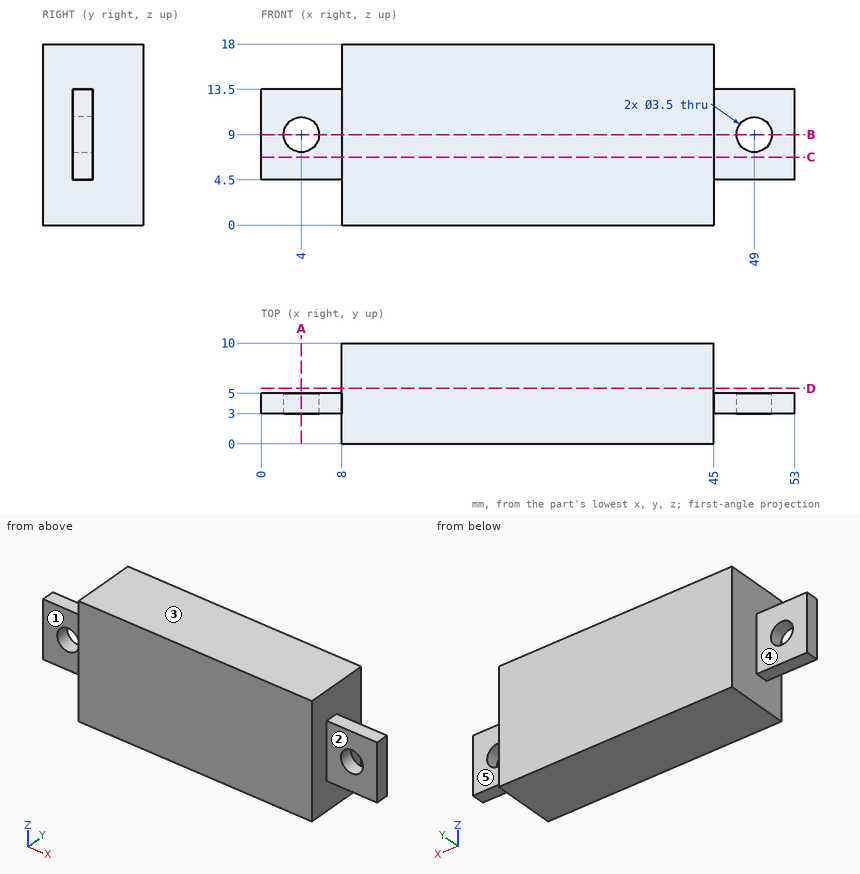
Check sheet for the drawn part. Datum: minimum x, y, z corner. Units: mm. A direction names the side the tool comes from. Give positions to 0.01 mm unless a question says otherwise; leave off trailing zeros. Loops run counter-clockwise (first coordinate to the right, second up) from the corner with the lowest first, then second, coordinate; pieces in that order, holes last.
1) Sectioned sample at A-A, the plane x = 4. Enter the section's corners in (y, z).
2) Depth check by flat-ended pin: pin 1 Ø5 at (y, z) = (3.5, 6) entering from -X; pin 2 Ø2 at (y, z) = (9, 13.5) entering from +X; pin 3 Ø1 at (x, y) = (50.5, 4.5) entering from +Z; pin 4 Ø0.6 at (x, y) = (49.5, 4.5) entering from -Z. Enter the tip coordinate at first touch or a pass-through.
3) Thickness scan on line 1 along X through (y, z) = (3.45, 9); line 2 along X through (y, z) = (5, 14); line 3 along Z through (x, y) = (6.5, 4). Record the ranges inside material, lowest first.
4) Set-up check for the marked faces 1, 2, 3, 4 and 5: record each of +Z, -Z, +X, -X, +Y, -Y from which the full face is reachable in a straight line by a thin tool's end or side.
5) Sectioned sample at B-B, the plane z = 9. Enter the section's corners in (x, y).
6) Sectioned sample at D-D, the plane y = 5.5. Enter the section's corners in (x, z), then the cut area to 3 significant figures.
7) Sectioned sample at C-C, the plane z = 6.75. Enter the section's corners in (x, y), then the cut area to 3 significant figures.
Answers:
1. outline: (3, 4.5) - (5, 4.5) - (5, 7.25) - (3, 7.25) - close; (3, 10.75) - (5, 10.75) - (5, 13.5) - (3, 13.5) - close
2. pin 1: stops at x = 0
2. pin 2: stops at x = 45
2. pin 3: stops at z = 13.5
2. pin 4: stops at z = 4.5
3. line 1: x = 0 to 2.25, 5.75 to 47.25, 50.75 to 53
3. line 2: x = 8 to 45
3. line 3: z = 4.5 to 13.5
4. face 1: +Z, -Z, -X, -Y
4. face 2: +Z, -Z, +X, -Y
4. face 3: +Z, +X, -X, +Y, -Y
4. face 4: +Z, -Z, -X, +Y
4. face 5: +Z, -Z, +X, +Y
5. outline: (0, 3) - (2.25, 3) - (2.25, 5) - (0, 5) - close; (5.75, 3) - (8, 3) - (8, 0) - (45, 0) - (45, 3) - (47.25, 3) - (47.25, 5) - (45, 5) - (45, 10) - (8, 10) - (8, 5) - (5.75, 5) - close; (50.75, 3) - (53, 3) - (53, 5) - (50.75, 5) - close
6. outline: (8, 0) - (45, 0) - (45, 18) - (8, 18) - close
6. area: 666 mm2
7. outline: (0, 3) - (8, 3) - (8, 0) - (45, 0) - (45, 3) - (53, 3) - (53, 5) - (45, 5) - (45, 10) - (8, 10) - (8, 5) - (0, 5) - close
7. area: 402 mm2
